Autodesk Inventor part; units mm, degrees
ref_plane "YZ Plane" through (0, 0, 0) normal (1, 0, 0) x (0, 1, 0)
ref_plane "XZ Plane" through (0, 0, 0) normal (0, 1, 0) x (-1, 0, 0)
ref_plane "XY Plane" through (0, 0, 0) normal (0, 0, 1) x (1, 0, 0)
sketch "スケッチ1" plane through (0, 0, 0) normal (0, 0, 1) x (1, 0, 0)
  circle A0 centre (13.0815, -13.0815) radius 1
  circle A1 centre (-13.0815, 13.0815) radius 1
  circle A2 centre (13.0815, 13.0815) radius 1
  line L0 (-17.5, -17.5) -> (17.5, -17.5)
  line L1 (17.5, -17.5) -> (17.5, -13.2)
  line L2 (17.5, 22) -> (-17.5, 22)
  line L3 (-17.5, 22) -> (-17.5, 13.2505)
  line L4 (-17.0382, 13.2505) -> (-17.5, 13.2505)
  line L5 (-17.5, 13.2505) -> (-17.5, 13.2)
  line L6 (-17.5, 10.2) -> (-17.0382, 10.2)
  line L7 (-17.0382, 10.2) -> (-17.0382, 13.2505)
  line L8 (-17, -10.2) -> (-17.5, -10.2)
  line L9 (-17.5, -10.2) -> (-17.5, -13.2)
  line L10 (-17.5, -13.2) -> (-17, -13.2)
  line L11 (-17, -13.2) -> (-17, -10.2)
  line L12 (17.5, -10.2) -> (17, -10.2)
  line L13 (17, -10.2) -> (17, -13.2)
  line L14 (17, -13.2) -> (17.5, -13.2)
  line L15 (17.5, -13.2) -> (17.5, -10.2)
  line L16 (17.5, 13.2) -> (17, 13.2)
  line L17 (17, 13.2) -> (17, 10.2)
  line L18 (17, 10.2) -> (17.5, 10.2)
  line L19 (17.5, 10.2) -> (17.5, 13.2)
  line L20 (17, 13.2) -> (17.5, 13.2)
  line L21 (17.5, 13.2) -> (17.5, 22)
  line L22 (17.5, 10.2) -> (17.5, 13.2)
  line L23 (17.5, -10.2) -> (17.5, 10.2)
  line L24 (17.5, -13.2) -> (17.5, -10.2)
  line L25 (-17.5, -13.2) -> (-17.5, -17.5)
  line L26 (-17.5, -10.2) -> (-17.5, -13.2)
  line L27 (-17.5, 13.2505) -> (-17.5, 13.2)
  line L28 (-17.5, 13.2) -> (-17.5, 10.2)
  line L29 (-17.5, 10.2) -> (-17.5, -10.2)
  line L30 (-17.5, 13.2) -> (-17.5, 10.2)
  circle A3 centre (-13.0815, 13.0815) radius 1
  circle A4 centre (13.0815, 13.0815) radius 1
  circle A5 centre (-13.0815, -13.0815) radius 1
  circle A6 centre (13.0815, -13.0815) radius 1
  circle A7 centre (-13.0815, -13.0815) radius 1
  point P0 (0, 0)
  point P1 (0, 0)
  dimension "d0" = 39.5
  dimension "d1" = 2
extrude "押し出し1" add sketch "スケッチ1" along normal blind 1 contours L25 L10 L11 L8 L29 L6 L7 L4 L3 L2 L21 L16 L17 L18 L23 L12 L13 L14 L1 L0
fillet "フィレット1" radius 1.5 4 edges at (-17.5, -17.5, 0.5) (-17.5, 22, 0.5) (17.5, 22, 0.5) (17.5, -17.5, 0.5)
sketch "スケッチ2" plane through (0, 0, 1) normal (0, 0, 1) x (1, 0, 0)
  line L0 (17.5, 20.5) -> (17.5, 13.2)
  line L1 (-16, 22) -> (16, 22)
  line L2 (-17.5, 13.2505) -> (-17.5, 20.5)
  line L3 (16, -17.5) -> (-16, -17.5)
  line L4 (17.5, 20) -> (-17.5, 20)
  line L5 (0, 22) -> (0, -17.5)
  point P0 (0, 0)
  point P1 (2.5, 20)
  point P2 (7.5, 20)
  point P3 (12.5, 20)
  point P4 (-2.5, 20)
  point P5 (-7.5, 20)
  point P6 (-12.5, 20)
  dimension "d5" = 2
  dimension "d6" = 12.5
  dimension "d9" = 5
  dimension "d10" = 5
hole "Hole1" at (2.5, 20, 1) at (7.5, 20, 1) at (12.5, 20, 1) at (-12.5, 20, 1) at (-7.5, 20, 1) at (-2.5, 20, 1) direction (0, 0, -1) diameter 1 end through all
sketch "スケッチ3" plane through (0, 0, 1) normal (0, 0, 1) x (1, 0, 0)
  circle A0 centre (-2.5, 20) radius 0.5
  circle A1 centre (-7.5, 20) radius 0.5
  circle A2 centre (-12.5, 20) radius 0.5
  circle A3 centre (12.5, 20) radius 0.5
  circle A4 centre (7.5, 20) radius 0.5
  circle A5 centre (2.5, 20) radius 0.5
  circle A6 centre (12.5, 20) radius 1.5
  circle A7 centre (7.5, 20) radius 1.5
  circle A8 centre (2.5, 20) radius 1.5
  circle A9 centre (-2.5, 20) radius 1.5
  circle A10 centre (-7.5, 20) radius 1.5
  circle A11 centre (-12.5, 20) radius 1.5
  point P0 (0, 0)
  dimension "d18" = 3
  dimension "d19" = 3
  dimension "d20" = 3
  dimension "d21" = 3
  dimension "d22" = 3
  dimension "d23" = 3
extrude "押し出し2" add sketch "スケッチ3" along normal blind 0.01
equation "\"d19\" = d18"
equation "\"d20\" = d18"
equation "\"d21\" = d18"
equation "\"d22\" = d18"
equation "\"d23\" = d18"
properties part number "SLIPRING_SRG-1-6G_"
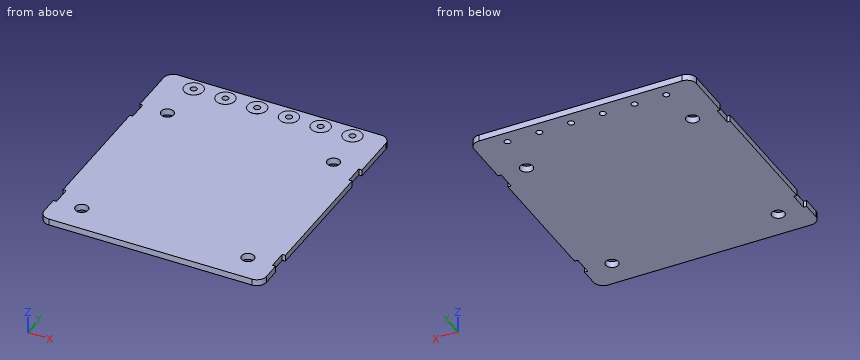
Check sheet for the modelled part. Datum: model origin and axes. Units: mm. Give positions to 0.01 mm unless a question says otherwise; leave off trailing zeros. Use CSV: the item, a comma, the result in double quotes. Start each with the question number.
1) Material ranges on line 1 (X direction, y = -13, z = 0.3); line 2 (Y direction, x = -2.5, z = 0.2); line 3 (Z direction, x = -3, y = -1.5), recorded low to high. Write a range as from..to.
2) Go/stop test with flat-tipped pins: P1, Ø12, axis at x = 10, y = -3, coming from the +Z side; P2, Ø0.6, axis at x = -17, z = 0.5, coming from the -Y side. Record where each tip stops, or that it passes through.
3) Sectioned sample at A-A, the plane z = 0.75. Give the number of separate pieces and of enclosed holes in the cut face, plus the area to 3 significant figures.
Recorded:
1,line 1,"-17..-14.08, -12.08..12.08, 14.08..17"
1,line 2,"-17.5..19.5, 20.5..22"
1,line 3,"0..1"
2,P1,"z = 1"
2,P2,"y = -17.33"
3,separate pieces,"1"
3,enclosed holes,"10"
3,area,"1,360 mm2"
